```python
from build123d import *

# Parameters (mm, degrees)
SKETCH1_W            = 40
SKETCH1_H            = 36
BODY_DEPTH           = 28
SENSOR_HOUSING_START = 28
SKETCH2_W            = 22
SKETCH2_H            = 20
SENSOR_HOUSING_DEPTH = 7
INLET_THREAD_START   = -31
SKETCH3_R            = 10.4775
INLET_THREAD_DEPTH   = 11
OUTLET_THREAD_START  = 20
SKETCH4_R            = 10.4775
OUTLET_THREAD_DEPTH  = 11
INLET_BORE_START     = -31
SKETCH5_R            = 4.5
INLET_BORE_DEPTH     = 8
OUTLET_BORE_START    = 23
SKETCH6_R            = 4.5
OUTLET_BORE_DEPTH    = 8
CABLE_STUB_START     = 10
SKETCH7_R            = 2
CABLE_STUB_DEPTH     = 15
FLOW_ARROW_START     = 18
FLOW_ARROW_DEPTH     = 0.6


with BuildPart() as part:
    # Sketch1 → Body (new body)
    with BuildSketch(Plane(origin=(0, 0, 0), x_dir=(1, 0, 0), z_dir=(0, 1, 0))):
        Rectangle(SKETCH1_W, SKETCH1_H)
    extrude(amount=BODY_DEPTH)

    # Sketch2 → Sensor_Housing (add)
    with BuildSketch(Plane(origin=(0, 0, 0), x_dir=(1, 0, 0), z_dir=(0, 1, 0)).offset(SENSOR_HOUSING_START)):
        Rectangle(SKETCH2_W, SKETCH2_H)
    extrude(amount=SENSOR_HOUSING_DEPTH)

    # Sketch3 → Inlet_Thread (add)
    with BuildSketch(Plane(origin=(0, 0, 0), x_dir=(0, 0, -1), z_dir=(1, 0, 0)).offset(INLET_THREAD_START)):
        with Locations((0, 15)):
            Circle(SKETCH3_R)
    extrude(amount=INLET_THREAD_DEPTH)

    # Sketch4 → Outlet_Thread (add)
    with BuildSketch(Plane(origin=(0, 0, 0), x_dir=(0, 0, -1), z_dir=(1, 0, 0)).offset(OUTLET_THREAD_START)):
        with Locations((0, 15)):
            Circle(SKETCH4_R)
    extrude(amount=OUTLET_THREAD_DEPTH)

    # Sketch5 → Inlet_Bore (cut)
    with BuildSketch(Plane(origin=(0, 0, 0), x_dir=(0, 0, -1), z_dir=(1, 0, 0)).offset(INLET_BORE_START)):
        with Locations((0, 15)):
            Circle(SKETCH5_R)
    extrude(amount=INLET_BORE_DEPTH, mode=Mode.SUBTRACT)

    # Sketch6 → Outlet_Bore (cut)
    with BuildSketch(Plane(origin=(0, 0, 0), x_dir=(0, 0, -1), z_dir=(1, 0, 0)).offset(OUTLET_BORE_START)):
        with Locations((0, 15)):
            Circle(SKETCH6_R)
    extrude(amount=OUTLET_BORE_DEPTH, mode=Mode.SUBTRACT)

    # Sketch7 → Cable_Stub (add)
    with BuildSketch(Plane.XY.offset(CABLE_STUB_START)):
        with Locations(Location((0, 31.5, 0), (0, 0, 180))):
            Circle(SKETCH7_R)
    extrude(amount=CABLE_STUB_DEPTH)

    # Sketch8 → Flow_Arrow (add)
    with BuildSketch(Plane.XY.offset(FLOW_ARROW_START)):
        Polygon((-12, 7), (6, 7), (6, 4), (13, 9), (6, 14), (6, 11), (-12, 11), align=None)
    extrude(amount=FLOW_ARROW_DEPTH)


solid = part.part
```
Verification items for the finished model (mm, model axes). A direction names the side the tool comes from. Coordinates: 2 decimals unless noted, no trailing zeros. Write each loop counter-clockwise with the first axis right and the second up, starting at its lowest first coordinate (ties: lowest second). Pieces come first, ordered by that corner, then holes. Notation, with made-up numbers: (21.5, -14) - (61.5, -14) arc R23 ccw to (61.5, 0) - close; hole circle Ø1 at (-4, 55.5). An arc over 180 degrees is marked (long way). Write item = value, one per line.
Q1. Cross-section at D-D (x = -3). Enter the section's corners in (y, z), plus the area to 3 significant figures.
Answer:
outline = (0, -18) - (28, -18) - (28, -10) - (35, -10) - (35, 10) - (28, 10) - (28, 18) - (11, 18) - (11, 18.6) - (7, 18.6) - (7, 18) - (0, 18) - close
area = 1,150 mm²
Q2. Cross-section at B-B (z = 13.5). Enter the section's corners in (x, y), plus the area to 3 significant figures.
Answer:
outline = (-20, 0) - (20, 0) - (20, 28) - (-20, 28) - close; circle Ø4 at (0, 31.5)
area = 1,130 mm²
Q3. Mould release check, pull along Y, two halves, no side actions. Record for faces 5 (the face through (23, 15, 0)), 6 (the face through (-11, 31, 0)), 7 (the face through (-25.577, 23.835, -5.633)): released by +Y, released by -Y, zero draft, split by the parting line, or undercut.
Answer:
face_5 = undercut
face_6 = zero draft
face_7 = split by the parting line
Q4. Cross-section at C-C (z = 0). Enter the section's corners in (x, y), plus the area to 3 significant figures.
Answer:
outline = (-31, 4.52) - (-20, 4.52) - (-20, 0) - (20, 0) - (20, 4.52) - (31, 4.52) - (31, 10.5) - (23, 10.5) - (23, 19.5) - (31, 19.5) - (31, 25.48) - (20, 25.48) - (20, 28) - (11, 28) - (11, 35) - (-11, 35) - (-11, 28) - (-20, 28) - (-20, 25.48) - (-31, 25.48) - (-31, 19.5) - (-23, 19.5) - (-23, 10.5) - (-31, 10.5) - close
area = 1,590 mm²
Q5. Go/stop test with flat-tipped pins: pin 1 Ø0.7 at (y, z) = (5.5, 18) entering from -X; pin 2 Ø8.5 at (x, y) = (-5.5, 15.5) entering from +Z; pin 3 Ø12 at (x, z) = (21, -0.5) entering from +Y. Record where each tip stops, or that it passes through.
Answer:
pin_1 = -20
pin_2 = 18
pin_3 = 28
Q6. Cross-section at A-A (y = 31.5). Enter the section's corners in (x, z), plus the area to 3 significant figures.
Answer:
outline = (-11, -10) - (11, -10) - (11, 10) - (2, 10) - (2, 25) - (-2, 25) - (-2, 10) - (-11, 10) - close
area = 500 mm²
Q7. Material ranges on L1, parallel to Y at x = 25, z = 0; L2, parallel to X at y = 12, z = -13.5; L3, parallel to Z at x = -7, y = 33, recorded low to high. Write a range as from..to.
Answer:
L1 = 4.52..10.5, 19.5..25.48
L2 = -20..20
L3 = -10..10
Q8. Access from +Z, -Z, +X, -X, +Y, -Y to the whole of each face (thin tool, end or side, straight path). Record for faces 1 (the face through (0, 9, 18.6)), 2 (the face through (-20, 4, 0)), 3 (the face through (0.434, 33.452, 17.395)), 4 (the face through (11, 31, 0)).
Answer:
face_1 = +Z, +X, -X, -Y
face_2 = -X
face_3 = +Z
face_4 = +Z, -Z, +X, +Y
